Could you check a few things on this model? Use its own coordinates, in mm. A direction names the side the tool comes from. Round coordinates to 2 decimals unless told otherwise and drop trailing zeros. Loops run counter-clockwise (first coordinate to the right, second up) from the corner with the lowest first, then second, coordinate; pieces in that order, holes last.
from build123d import *
from OCP.BRepFilletAPI import BRepFilletAPI_MakeChamfer

# Parameters (mm, degrees)
SKETCH1_R           = 5.75
BOSS_EXTRUDE1_DEPTH = 3
BOSS_EXTRUDE2_DEPTH = 0.15
CIRPATTERN1_COUNT   = 2
SKETCH4_R           = 2.5
CUT_EXTRUDE1_DEPTH  = 65.299031318
CHAMFER1_SIZE       = 1
CHAMFER1_SIZE2      = 1.191753593


with BuildPart() as part:
    # Sketch1 → Boss-Extrude1 (new, symmetric)
    with BuildSketch(Plane(origin=(0, 0, 0), x_dir=(1, 0, 0), z_dir=(0, 1, 0))):
        with Locations(Location((0, 0, 0), (0, 0, 270))):
            Circle(SKETCH1_R)
    extrude(amount=BOSS_EXTRUDE1_DEPTH, both=True)

    # Sketch3 → Boss-Extrude2 (add, symmetric)
    with BuildSketch(Plane(origin=(0, 0, 0), x_dir=(0.9743700647852351, -0.22495105434386548, 0), z_dir=(-0.2249510543438655, -0.9743700647852352, 0))):
        with BuildLine():
            Line((-4.454728917, 2.312449404), (-8.310390593, 4.705233436))
            Line((-8.310390593, 4.705233436), (-8.310390593, 60.5))
            ThreePointArc((-8.310390593, 60.5), (-7.431710937, 62.621320344), (-5.310390593, 63.5))
            Line((-5.310390593, 63.5), (-2.961672938, 63.5))
            ThreePointArc((-2.961672938, 63.5), (0.007877818, 62.522656871), (1.816520564, 59.972707322))
            add(Edge.make_bspline(
                [(1.816520564, 59.972707322), (11.305446488, 30.906067871), (5.007624384, 0.848133108)],
                knots=[0, 0, 0, 1, 1, 1], degree=2))
            add(Edge.make_bspline(
                [(-4.454728917, 2.312449404), (0.194469727, 8.941584866), (5.007624384, 0.848133108)],
                knots=[0, 0, 0, 1, 1, 1], degree=2))
        make_face()
    boss_extrude2 = extrude(amount=BOSS_EXTRUDE2_DEPTH, both=True)

    # CirPattern1: Boss-Extrude2 ×2 about axis
    cirpattern1_axis = Axis((0, -3, 0), (0, 1, 0))
    for i in range(1, CIRPATTERN1_COUNT):
        add(boss_extrude2.rotate(cirpattern1_axis, i * 360 / CIRPATTERN1_COUNT))

    # Sketch4 → Cut-Extrude1 (cut, through all)
    with BuildSketch(Plane(origin=(0, 3, 0), x_dir=(1, 0, 0), z_dir=(0, 1, 0))):
        with Locations(Location((0, 0, 0), (0, 0, 270))):
            Circle(SKETCH4_R)
    extrude(amount=-CUT_EXTRUDE1_DEPTH, mode=Mode.SUBTRACT)

    # Chamfer1: one chamfer whose edges measure the first distance from different faces: ONE call of the kernel's chamfer builder (chamfer() names one face for all edges)
    chamfer1_edges_1 = [part.edges().sort_by_distance(p)[0] for p in [
        (0, -3, -2.5),
    ]]
    chamfer1_side_1 = [part.faces().sort_by_distance(p)[0] for p in [
        (0, 0, -2.5),
    ]]
    chamfer1_edges_2 = [part.edges().sort_by_distance(p)[0] for p in [
        (0, 3, -2.5),
    ]]
    chamfer1_side_2 = [part.faces().sort_by_distance(p)[0] for p in [
        (0, 3, -5.58736544),
    ]]
    chamfer1 = BRepFilletAPI_MakeChamfer(part.part.solid().wrapped)
    for e in chamfer1_edges_1:
        chamfer1.Add(CHAMFER1_SIZE, CHAMFER1_SIZE2, e.wrapped, chamfer1_side_1[0].wrapped)  # the first distance lies on this face
    for e in chamfer1_edges_2:
        chamfer1.Add(CHAMFER1_SIZE, CHAMFER1_SIZE2, e.wrapped, chamfer1_side_2[0].wrapped)  # the first distance lies on this face
    add(Compound.cast(chamfer1.Shape()), mode=Mode.REPLACE)


solid = part.part
Item 1: If I drill on line 1 along X through (y, z) = (0.85, 0); line 2 along Z through (x, y) = (2.25, -1); line 3 along Y through (x, z) = (-5, -26), over which ranges is the centre line in solid material (lowest first)?
Results list:
line 1: x = -5.75 to -2.5, 2.5 to 5.75
line 2: z = -5.29 to -1.09, 1.09 to 5.29
line 3: y = -1.31 to -1
Item 2: We'd pull the mould along X, two halves only. Please class faces 3 (the cylindrical face through (-2.44, -0.07, -0.54)), 4 (the flat face through (-4, -3, 0)): released by +X, released by -X, zero draft, split by the parting line, or undercut.
Results list:
face 3: undercut
face 4: zero draft
Item 3: Will these pins go through, and if not, where does the flat tip stop? pin 1 (6 mm diameter, centred on x = 0, z = 0, fed in from -Y); pin 2 (6 mm diameter, centred on x = -2, z = 24.5, fed in from -Y); pin 3 (1 mm diameter, centred on x = -3.5, z = 37.5, fed in from +Y).
Results list:
pin 1: stops at y = -2.42
pin 2: stops at y = -0.38
pin 3: stops at y = 1.08
Item 4: If we section it at A-A, the plane z = 0: Please give me the cut outline in (x, y).
Results list:
outline: (-5.75, -3) - (-3.69, -3) - (-2.5, -2) - (-2.5, 1.81) - (-3.5, 3) - (-5.75, 3) - close; (2.5, -2) - (3.69, -3) - (5.75, -3) - (5.75, 3) - (3.5, 3) - (2.5, 1.81) - close
Item 5: For faces 1 (the flat face through (0, 3, 4)), 2 (the cylindrical face through (1.727, 0.042, 5.484)), which set-ups out of +Z, -Z, +X, -X, +Y, -Y let a thin tool reach every point of the face, with its end or its side?
Results list:
face 1: +Z, -Z, +X, -X, +Y
face 2: none
